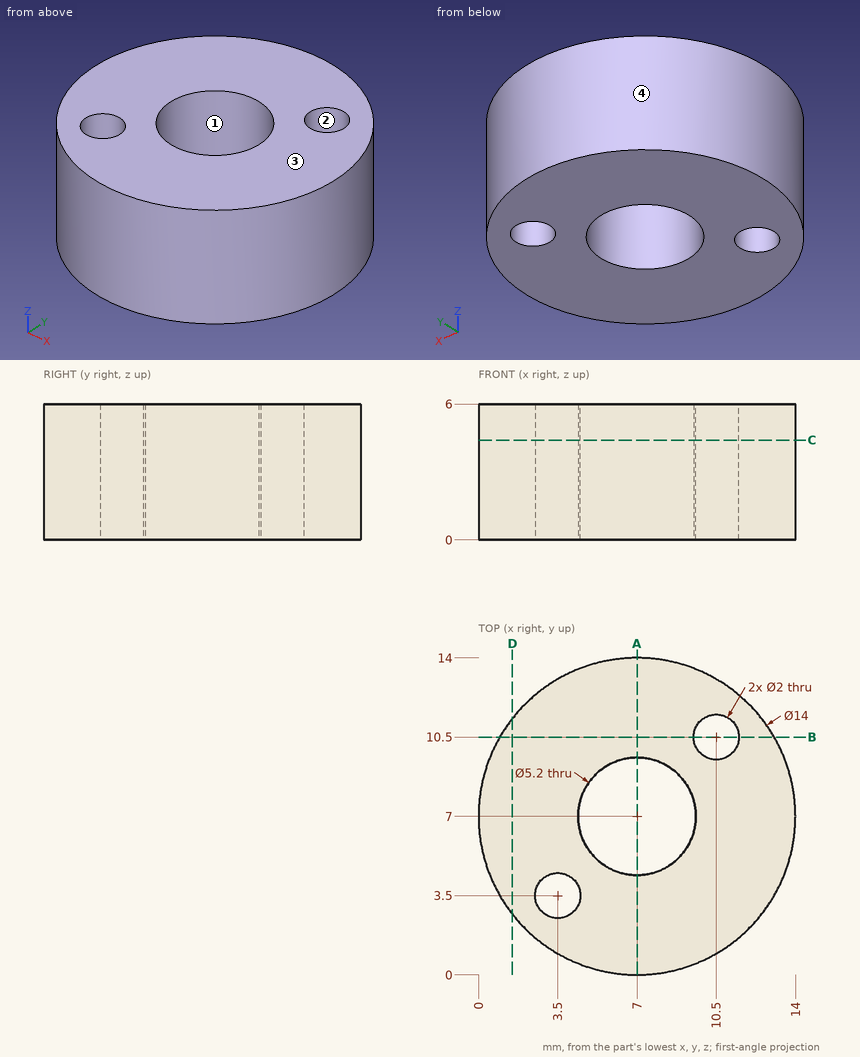
Can you work these out from the drawing? Everything is in mm from the part's minimum corner. Give positions to 0.01 mm unless a question says otherwise; leave off trailing zeros. Loops run counter-clockwise (first coordinate to the right, second up) from the corner with the lowest first, then second, coordinate; pieces in that order, holes last. Notation, with made-up numbers: M -27,77.5 L 8,77.5 A28 ccw 8,112.5 Z; hole C -26.5,-2 d9. An arc over 180 degrees is marked long. Use CSV: the item, a comma, the result in double quotes. Start each with the question number.
1. Imagine slicing it at D-D, the plane x = 1.5. Write out the boundary of the cut face in (y, z), plus the area to 3 significant figures.
2. Imagine slicing it at C-C, the plane z = 4.4. Write out the boundary of the cut face in (x, y).
3. Imagine slicing it at A-A, the plane x = 7. Write out the boundary of the cut face in (y, z), plus the area to 3 significant figures.
4. Imagine slicing it at B-B, the plane y = 10.5. Write out the boundary of the cut face in (x, z), plus the area to 3 significant figures.
5. If we mould it in two halves opening along X, with no side actions, what happens to the marked faces 1, 2, 3 and 4? For each: released by +X, released by -X, zero draft, split by the parting line, or undercut.
6. For P1, Ø1, axis at x = 6, y = 8, coming from the -Z side; P2, Ø1, axis at x = 3.5, z = 4, coming from the +Y side, each with a flat end and sliding along its axis, tell me the tip position at first contact or that it passes through.
7. If I drill on L1, parallel to Y at x = 7, z = 3.9; L2, parallel to Y at x = 3.5, z = 0.9, over which ranges is the centre line in solid material (lowest first)?
Response values:
1,outline,"M 2.67,0 L 11.33,0 L 11.33,6 L 2.67,6 Z"
1,area,"52.0 mm^2"
2,outline,"C 7,7 d14; hole C 3.5,3.5 d2; hole C 7,7 d5.2; hole C 10.5,10.5 d2"
3,outline,"M 0,0 L 4.4,0 L 4.4,6 L 0,6 Z; M 9.6,0 L 14,0 L 14,6 L 9.6,6 Z"
3,area,"52.8 mm^2"
4,outline,"M 0.94,0 L 9.5,0 L 9.5,6 L 0.94,6 Z; M 11.5,0 L 13.06,0 L 13.06,6 L 11.5,6 Z"
4,area,"60.7 mm^2"
5,face 1,"undercut"
5,face 2,"undercut"
5,face 3,"zero draft"
5,face 4,"split by the parting line"
6,P1,"through"
6,P2,"y = 13.32"
7,L1,"0 to 4.4, 9.6 to 14"
7,L2,"0.94 to 2.5, 4.5 to 13.06"
